Read the model definition and answer for the solid it produces. Units are mm, in the model's axes. A direction names the side the tool comes from. Round coordinates to 2 decimals unless told otherwise and drop trailing zeros. Order: outer loops, then holes, each group sorted by start corner. A loop starts at its lowest first (then second) coordinate and runs counter-clockwise, first axis right, second up. Notation, with made-up numbers: (43.25, 83.5) -> (95.25, 83.5) arc R12 cw to (95.25, 96.5) -> close; hole circle Ø9 at (64, 47). An arc over 180 degrees is marked (long way). One line per item, written item: value. Start each with the question number.
1. Section A-A (y = 10) is taken. State how many separate pieces and enclosed holes the cut face has, then the cut area to 3 significant figures.
2. Flat-ended cylindrical pins translate along their axes: pin 1 Ø1.5 at (x, y) = (44.5, -25) entering from +Z; pin 2 Ø10 at (y, z) = (13, 47.5) entering from -X; pin 3 Ø3 at (x, y) = (84.5, 45.5) entering from -Z. Find the tip coordinate at first contact, or state that the pin passes through.
3. For faces 5 (the face through (-50, -4, 50)), 6 (the face through (-50, -4, 147)), 7 (the face through (-54.1, -0.3, 142.7)), 8 (the face through (82.28, -13.375, 140.472)), 9 (the face through (-49.352, 2.172, 99.179)), determine the directions among +Z, -Z, +X, -X, +Y, -Y from which every point of the face is accessible in a straight line to the end or side of a thin tool.
4. Consider line 1 (Z direction, x = 55, y = -0.5); line 2 (Z direction, x = -10, y = -54.5); line 3 (Y direction, x = 55, z = 98). Determine where each line is inside the solid, lowest interval first.
5. The mould has two halves that part along Y. Classify faces 1 (the face through (56.543, -7.424, 24.65)), 2 (the face through (-41, 41, 0)), 3 (the face through (-59.85, -13.29, 26.77)), 4 (the face through (62, -40, 101)): released by +Y, released by -Y, zero draft, split by the parting line, or undercut.
6. Section B-B (x = 88) is taken. Give the vertices of the cut face in (y, z) (3 decimals), then the cut area to 3 significant figures.
7. Section C-C (z = 24.5) is taken. Give the vertices of the cut face in (x, y), then the cut area to 3 significant figures.
Autodesk Inventor part; units mm, degrees
ref_plane "YZ Plane" through (0, 0, 0) normal (1, 0, 0) x (0, 1, 0)
ref_plane "XZ Plane" through (0, 0, 0) normal (0, 1, 0) x (-1, 0, 0)
ref_plane "XY Plane" through (0, 0, 0) normal (0, 0, 1) x (1, 0, 0)
sketch "Sketch1" plane through (0, 0, 0) normal (1, 0, 0) x (0, 1, 0)
  line L0 (0, 0) -> (61.5752, 0)
  line L1 (61.5752, 0) -> (61.0322, 54.3)
  line L2 (0, 197) -> (0, 0)
  line L3 (56.775, 50) -> (57.275, 0)
  line L4 (53.9, 54.3) -> (53.9, 142.7)
  line L5 (0, 54.3) -> (61.0322, 54.3)
  line L6 (56.775, 50) -> (0, 50)
  line L7 (0, 98.5) -> (53.9, 98.5) construction
  line L8 (0, 197) -> (61.5752, 197)
  line L9 (61.5752, 197) -> (61.0322, 142.7)
  line L10 (56.775, 147) -> (57.275, 197)
  line L11 (0, 142.7) -> (61.0322, 142.7)
  line L12 (56.775, 147) -> (0, 147)
  line L13 (0, 142.7) -> (0, 54.3)
  dimension "d0" = 114.55
  dimension "d3" = 113.55
  dimension "d4" = 107.8
  dimension "d5" = 4.3
  dimension "d8" = 50
  dimension "d9" = 4.3
  dimension "d25" = 197
revolve "Revolution1" add sketch "Sketch1" angle 360 about axis through (0, 0, 197) along (0, 0, -1) contours L3 L6 L2 L5 L1 L0 | L2 L11 L4 L5 | L2 L12 L10 L8 L9 L11
sketch "Sketch2" plane through (0, 0, 0) normal (0, 1, 0) x (-1, 0, 0)
  line L0 (-57.275, 0) -> (57.275, 0)
  line L1 (0, 197) -> (0, 0)
  line L2 (0, 98) -> (-102, 98)
  line L3 (-102, 98) -> (-102, 146.1252)
  line L4 (-102, 146.1252) -> (-58.6, 145.6912)
  line L5 (-58.6, 145.6912) -> (-58.6, 98)
  line L6 (-62, 145.7252) -> (-62, 98)
  line L7 (0, 140.2) -> (-58.6, 140.2)
  line L8 (-62, 142.325) -> (-102, 142.725)
  line L9 (-57.275, 197) -> (57.275, 197)
  dimension "d10" = 98
  dimension "d13" = 102
  dimension "d14" = 89.45
  dimension "d15" = 88.65
  dimension "d16" = 84.4
  dimension "d17" = 40
  dimension "d18" = 3.4
  dimension "d19" = 3.4
revolve "Revolution2" add sketch "Sketch2" angle 360 about axis through (0, 0, 98) along (1, 0, 0) contours L1 L2 L5 L7 | L5 L2 L6 L4 | L6 L8 L3 L4
sketch "Sketch3" plane through (0, 0, 147) normal (0, 0, 1) x (1, 0, 0)
  circle A0 centre (0, 0) radius 56.775
  circle A1 centre (0, 0) radius 49.4
  dimension "d26" = 98.8
extrude "Extrusion1" cut sketch "Sketch3" against normal through all contours A1
sketch "Sketch4" plane through (62, 0, 98) normal (1, 0, 0) x (0, 0, -1)
  circle A0 centre (0, 0) radius 38.6
  circle A1 centre (0, 0) radius 44.325
  dimension "d23" = 77.2
extrude "Extrusion2" cut sketch "Sketch4" against normal up to surface contours A0
equation "\"d26\" = d1"
equation "\"d23\" = d2"
equation "\"d0\" = d11"
equation "\"d3\" = d21"
equation "\"d4\" = d1 + 2 * t11"
equation "\"d5\" = t21"
equation "\"d8\" = l11"
equation "\"d9\" = t21"
equation "\"d25\" = L1 + L2"
equation "\"d10\" = L1"
equation "\"d13\" = L3"
equation "\"d14\" = d12"
equation "\"d15\" = d22"
equation "\"d16\" = d2 + 2 * t12"
equation "\"d17\" = l12"
equation "\"d18\" = t22"
equation "\"d19\" = t22"
equation "\"d1\" = 98.8"
equation "\"d11\" = 114.55"
equation "\"d21\" = 113.55"
equation "\"l11\" = 50"
equation "\"L1\" = 98"
equation "\"L2\" = 99"
equation "\"L3\" = 102"
equation "\"t11\" = 4.5"
equation "\"t21\" = 4.3"
equation "\"Z1\" = 48"
equation "\"Z2\" = 49"
equation "\"Z3\" = 62"
equation "\"d2\" = 77.2"
equation "\"d12\" = 89.45"
equation "\"d22\" = 88.65"
equation "\"l12\" = 40"
equation "\"t12\" = 3.6"
equation "\"t22\" = 3.4"
equation "\"d7\" = t21"
equation "\"Size_Designation\" = 1.2345"
properties part number "JIS K 6739 90 Deg Lateral Reducer (DT) 100 x 100 x 75" material "PVC, Unplasticized"
Answer:
1. separate pieces: 3
1. enclosed holes: 2
1. area: 1,920 mm^2
2. pin 1: z = 147
2. pin 2: x = -60.58
2. pin 3: z = 78.94
3. face 5: -Z
3. face 6: +Z
3. face 7: none
3. face 8: +X
3. face 9: +Z, -Z
4. line 1: 50 to 54.3, 55.8 to 59.4, 136.6 to 140.2, 142.7 to 147
4. line 2: 50 to 54.3, 142.7 to 147
4. line 3: -42.2 to -38.6, 38.6 to 42.2
5. face 1: undercut
5. face 2: zero draft
5. face 3: split by the parting line
5. face 4: undercut
6. outline: circle Ø95.97 at (0, 98); hole circle Ø89.17 at (0, 98)
6. area: 989 mm^2
7. outline: circle Ø122.66 at (0, 0); hole circle Ø114.06 at (0, 0)
7. area: 1,600 mm^2
